from build123d import *

# Parameters (mm, degrees)
CROQUIS2_W              = 25.4
CROQUIS2_H              = 25.4
SALIENTE_EXTRUIR1_DEPTH = 210
CROQUIS3_R              = 5.765627546
CORTAR_EXTRUIR1_DEPTH   = 212.911420174


with BuildPart() as part:
    # Croquis2 → Saliente-Extruir1 (new, symmetric)
    with BuildSketch(Plane(origin=(0, 0, 0), x_dir=(0, 0, -1), z_dir=(1, 0, 0))):
        Rectangle(CROQUIS2_W, CROQUIS2_H)
    extrude(amount=SALIENTE_EXTRUIR1_DEPTH, both=True)

    # Croquis3 → Cortar-Extruir1 (cut, through all)
    with BuildSketch(Plane(origin=(0, 12.7, 0), x_dir=(1, 0, 0), z_dir=(0, 1, 0))):
        with Locations(Location((121.805313166, 0, 0), (0, 0, 270))):
            Circle(CROQUIS3_R)
        with Locations(Location((188.504509996, 0, 0), (0, 0, 270))):
            Circle(CROQUIS3_R)
        with BuildLine():
            Line((-180.393059191, 6.35), (-132.233607082, 6.35))
            ThreePointArc((-132.233607082, 6.35), (-125.883607082, 0), (-132.233607082, -6.35))
            Line((-132.233607082, -6.35), (-180.393059191, -6.35))
            ThreePointArc((-180.393059191, -6.35), (-186.743059191, 0), (-180.393059191, 6.35))
        make_face()
        with BuildLine():
            Line((19.606940809, 6.35), (67.766392918, 6.35))
            ThreePointArc((67.766392918, 6.35), (74.116392918, 0), (67.766392918, -6.35))
            Line((67.766392918, -6.35), (19.606940809, -6.35))
            ThreePointArc((19.606940809, -6.35), (13.256940809, 0), (19.606940809, 6.35))
        make_face()
    extrude(amount=-CORTAR_EXTRUIR1_DEPTH, mode=Mode.SUBTRACT)


solid = part.part
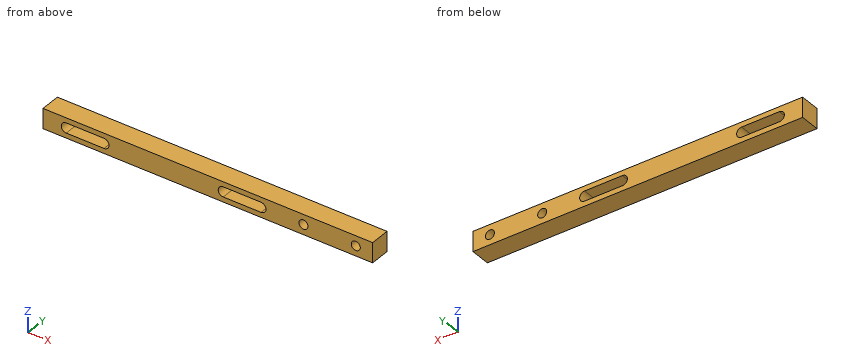
Part model, mm, in its own coordinate system. Coordinates: 2 decimals unless noted, no trailing zeros. Loops run counter-clockwise (first coordinate to the right, second up) from the corner with the lowest first, then second, coordinate; pieces in that order, holes last. Notation, with made-up numbers: (69.5, -27) - (117.5, -27) arc R17 ccw to (117.5, -16) - close; hole circle Ø8 at (77.5, -37). An arc over 180 degrees is marked (long way). Write each question's results on one line, items separated by ' | '. Start each with the question number.
Q1. Slice it at A-A on z = 0. Give the cut face in (x, y), and give its area (3 significant figures).
Q2. Slice it at C-C on y = -4.75. Give the cut face in (x, z).
Q3. Drop a flat-ended pin along its axis: pin 1 Ø13.5 at (x, z) = (121.81, 0) entering from +Y. Give the stop position or say it passes through.
Q4. Probe line 1 along X through (y, z) = (-5.75, 0); line 2 along Z through (x, y) = (21, -5.5); line 3 along Z through (x, y) = (123.5, -8). List the from-to ranges inside material, lowest first.
Q5. Slice it at B-B on x = 30. Give the cut face in (y, z), and give its area (3 significant figures).
Answer:
1) outline: (-210, -12.7) - (-186.74, -12.7) - (-186.74, 12.7) - (-210, 12.7) - close; (-125.88, -12.7) - (13.26, -12.7) - (13.26, 12.7) - (-125.88, 12.7) - close; (74.12, -12.7) - (116.04, -12.7) - (116.04, 12.7) - (74.12, 12.7) - close; (127.57, -12.7) - (182.74, -12.7) - (182.74, 12.7) - (127.57, 12.7) - close; (194.27, -12.7) - (210, -12.7) - (210, 12.7) - (194.27, 12.7) - close | area: 6,990 mm2
2) outline: (-210, -12.7) - (210, -12.7) - (210, 12.7) - (-210, 12.7) - close; hole (-180.39, -6.35) - (-132.23, -6.35) arc R6.35 ccw to (-132.23, 6.35) - (-180.39, 6.35) arc R6.35 ccw to start; hole (19.61, -6.35) - (67.77, -6.35) arc R6.35 ccw to (67.77, 6.35) - (19.61, 6.35) arc R6.35 ccw to start; hole circle Ø11.53 at (121.81, 0); hole circle Ø11.53 at (188.5, 0)
3) pin 1: stops at y = 12.7
4) line 1: x = -210 to -186.74, -125.88 to 13.26, 74.12 to 116.04, 127.57 to 182.74, 194.27 to 210 | line 2: z = -12.7 to -6.35, 6.35 to 12.7 | line 3: z = -12.7 to -5.51, 5.51 to 12.7
5) outline: (-12.7, -12.7) - (12.7, -12.7) - (12.7, -6.35) - (-12.7, -6.35) - close; (-12.7, 6.35) - (12.7, 6.35) - (12.7, 12.7) - (-12.7, 12.7) - close | area: 323 mm2
